from build123d import *

# Parameters (mm, degrees)
SKETCH_1_R          = 5
EXTRUDE_1_DEPTH     = 2.6
CHAMFER_1_SIZE      = 2.5
CUT_EXTRUDE_1_DEPTH = 0.95
SKETCH_3_R          = 2.5
EXTRUDE_2_DEPTH     = 37.4
CHAMFER_2_SIZE      = 0.2


with BuildPart() as part:
    # 草图1 → 凸台-拉伸1 (new body)
    with BuildSketch(Plane(origin=(0, 0, 0), x_dir=(1, 0, 0), z_dir=(0, 1, 0))):
        with Locations(Location((0, 0, 0), (0, 0, 270))):
            Circle(SKETCH_1_R)
    extrude(amount=EXTRUDE_1_DEPTH)

    # 倒角1
    chamfer_1_edges = [part.edges().sort_by_distance(p)[0] for p in [
        (0, 2.6, -5),
    ]]
    chamfer(chamfer_1_edges, length=CHAMFER_1_SIZE)

    # 草图2 → 切除-拉伸1 (cut)
    with BuildSketch(Plane.XZ):
        Polygon((1.54, -0.889119415), (1.54, 0.889119415), (0, 1.778238829), (-1.54, 0.889119415), (-1.54, -0.889119415), (0, -1.778238829), align=None)
    extrude(amount=-CUT_EXTRUDE_1_DEPTH, mode=Mode.SUBTRACT)

    # 草图3 → 凸台-拉伸2 (add)
    with BuildSketch(Plane(origin=(0, 2.6, 0), x_dir=(1, 0, 0), z_dir=(0, 1, 0))):
        with Locations(Location((0, 0, 0), (0, 0, 270))):
            Circle(SKETCH_3_R)
    extrude(amount=EXTRUDE_2_DEPTH)

    # 倒角2
    chamfer_2_edges = [part.edges().sort_by_distance(p)[0] for p in [
        (0, 40, -2.5),
    ]]
    chamfer(chamfer_2_edges, length=CHAMFER_2_SIZE)


solid = part.part
The listing builds one solid part. Answer for the finished solid, in the listing's coordinates (mm). A direction names the side the tool comes from. Coordinates: 2 decimals unless noted, no trailing zeros. Write each loop counter-clockwise with the first axis right and the second up, starting at its lowest first coordinate (ties: lowest second). Pieces come first, ordered by that corner, then holes. Notation, with made-up numbers: M 67.25,-25.5 L 125.25,-25.5 A26 cw 125.25,5.5 Z; hole C 74,62.5 d6. An arc over 180 degrees is marked long. Put each result on its own line as item: value. Start each with the question number.
1. A cutting plane is placed at A-A on z = 0. Write down the section's boundary in (x, y), then the cut area to 3 significant figures.
2. For a pull along Z with two mould halves and no side action, classify faces 1 (the flat face through (-1.54, 0.5, 0)), 2 (the flat face through (0, 40, 0)), 3 (the cylindrical face through (-2.44, 20.94, -0.54)) as pulls with the +Z half, pulls with the -Z half, needs draft (parallel to the pull), parting line crosses it, or undercut.
3. Consider line 1 (Y direction, x = 0.5, z = 1.25); line 2 (Z direction, x = -1.75, y = 18); line 3 (X direction, y = 20.5, z = -1). Determine where each line is inside the solid, lowest interval first. Write a range as from..to.
4. Which of the six approach directions +Z, -Z, +X, -X, +Y, -Y give full straight-line access (tool end or side, diameter ignored) to faces 4 (the conical face through (-1.595, 2.479, -2.08)), 5 (the flat face through (1.54, 0.5, 0))?
5. A cutting plane is placed at B-B on y = 7.5. Write down the section's boundary in (x, z), then the cut area to 3 significant figures.
6. Flat-ended cylindrical pins translate along their axes: P1, Ø1, axis at x = 3, z = -3.5, coming from the +Y side; P2, Ø4, axis at y = 19.5, z = -2, coming from the +X side; P3, Ø1.5, axis at x = -0.5, z = -0.5, coming from the -Y side. Find the tip coordinate at first contact, or state that the pin passes through.
Resolved:
1. outline: M -5,0 L -1.54,0 L -1.54,0.95 L 1.54,0.95 L 1.54,0 L 5,0 L 5,0.1 L 2.5,2.6 L 2.5,39.8 L 2.3,40 L -2.3,40 L -2.5,39.8 L -2.5,2.6 L -5,0.1 Z
1. area: 204 mm2
2. face 1: undercut
2. face 2: needs draft
2. face 3: parting line crosses it
3. line 1: y = 0.95..40
3. line 2: z = -1.79..1.79
3. line 3: x = -2.29..2.29
4. face 4: +Y
4. face 5: -Y
5. outline: C 0,0 d5
5. area: 19.6 mm2
6. P1: stops at y = 0.99
6. P2: stops at x = 2.5
6. P3: stops at y = 0.95
